from build123d import *

# Parameters (mm, degrees)
SKETCH1_R           = 1.3
BOSS_EXTRUDE1_DEPTH = 7.7
SKETCH2_R           = 1
CUT_EXTRUDE1_DEPTH  = 7.2
CUT_EXTRUDE2_REACH  = 9.7
SKETCH3_R           = 0.5


with BuildPart() as part:
    # Sketch1 → Boss-Extrude1 (new body)
    with BuildSketch(Plane(origin=(0, 0, 0), x_dir=(1, 0, 0), z_dir=(0, 1, 0))):
        Circle(SKETCH1_R)
    extrude(amount=BOSS_EXTRUDE1_DEPTH)

    # Sketch2 → Cut-Extrude1 (cut)
    with BuildSketch(Plane(origin=(0, 7.7, 0), x_dir=(1, 0, 0), z_dir=(0, 1, 0))):
        Circle(SKETCH2_R)
    extrude(amount=-CUT_EXTRUDE1_DEPTH, mode=Mode.SUBTRACT)

    # Sketch3 → Cut-Extrude2 (cut, up to next)
    with BuildSketch(Plane.XZ, mode=Mode.PRIVATE) as cut_extrude2_sk1:
        Circle(SKETCH3_R)
    cut_extrude2_tool1 = extrude(cut_extrude2_sk1.sketch, amount=-CUT_EXTRUDE2_REACH, mode=Mode.PRIVATE) & part.part
    add(cut_extrude2_tool1.solids().sort_by_distance((0, 0, 0))[0], mode=Mode.SUBTRACT)


solid = part.part
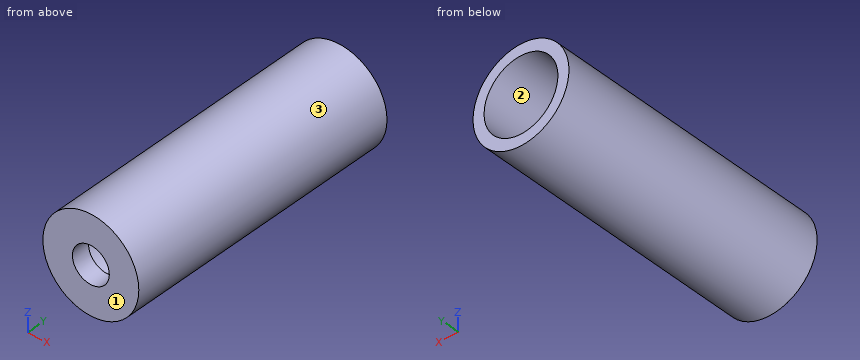
Verification items for the finished model (mm, model axes). Face numbers are marked on the shaded views. Coordinates: 2 decimals unless noted, no trailing zeros. Order: outer loops, then holes, each group sorted by start corner. A loop starts at its lowest first (then second) coordinate and runs counter-clockwise, first axis right, second up. Notation, with made-up numbers: M 8.25,-2 L 43.25,-2 A20 cw 43.25,15 Z; hole C 10,-12 d7. An arc over 180 degrees is marked long. One line per item, written item: value. Start each with the question number.
Item 1: Mould release check, pull along X, two halves, no side actions. Record for the marked faces 1, 2 and 3: pulls with the +X half, pulls with the -X half, needs draft (parallel to the pull), parting line crosses it, or undercut.
Item 2: Sectioned sample at D-D on x = -0.75. Record the cut outline in (y, z).
Item 3: Sectioned sample at B-B on x = 0. Record the cut outline in (y, z).
Item 4: Thickness scan on probe 1 along Z at (x, y) = (0, 0.45); probe 2 along Z at (x, y) = (0.05, 7.5). Record the ranges inside material, lowest first.
Item 5: Sectioned sample at C-C on y = 3.75. Record the cut outline in (x, z).
Item 6: Depth check by flat-ended pin: P1, Ø1.5, axis at x = 1, y = 1.5, coming from the +Z side; P2, Ø1.2, axis at x = 0, z = 0, coming from the +Y side; P3, Ø1, axis at y = 3, z = 1, coming from the -X side. Enter the tip coordinate at first touch or a pass-through.
Item 7: Sectioned sample at A-A on z = 0. Record the cut outline in (x, y).
Calculated:
1. face 1: needs draft
1. face 2: undercut
1. face 3: parting line crosses it
2. outline: M 0,-1.06 L 7.7,-1.06 L 7.7,-0.66 L 0.5,-0.66 L 0.5,0.66 L 7.7,0.66 L 7.7,1.06 L 0,1.06 Z
3. outline: M 0,-1.3 L 7.7,-1.3 L 7.7,-1 L 0.5,-1 L 0.5,-0.5 L 0,-0.5 Z; M 0,0.5 L 0.5,0.5 L 0.5,1 L 7.7,1 L 7.7,1.3 L 0,1.3 Z
4. probe 1: -1.3 to -0.5, 0.5 to 1.3
4. probe 2: -1.3 to -1, 1 to 1.3
5. outline: C 0,0 d2.6; hole C 0,0 d2
6. P1: z = 1.28
6. P2: y = 0.5
6. P3: x = -1.2
7. outline: M -1.3,0 L -0.5,0 L -0.5,0.5 L -1,0.5 L -1,7.7 L -1.3,7.7 Z; M 0.5,0 L 1.3,0 L 1.3,7.7 L 1,7.7 L 1,0.5 L 0.5,0.5 Z
